from build123d import *

# Parameters (mm, degrees)
SKIZZE1_W                       = 60
SKIZZE1_H                       = 60
AUFSATZ_LINEAR_AUSTRAGEN1_DEPTH = 3
VERRUNDUNG1_R                   = 3
SKIZZE2_R                       = 1.75
SKIZZE2_R_2                     = 3.25
SKIZZE2_R_3                     = 15
SCHNITT_LINEAR_AUSTRAGEN1_DEPTH = 12


with BuildPart() as part:
    # Skizze1 → Aufsatz-Linear austragen1 (new body)
    with BuildSketch(Plane.XY):
        Rectangle(SKIZZE1_W, SKIZZE1_H)
    extrude(amount=AUFSATZ_LINEAR_AUSTRAGEN1_DEPTH)

    # Verrundung1
    verrundung1_edges = [part.edges().sort_by_distance(p)[0] for p in [
        (-30, 30, 1.5),
        (30, 30, 1.5),
        (30, -30, 1.5),
        (-30, -30, 1.5),
    ]]
    fillet(verrundung1_edges, radius=VERRUNDUNG1_R)

    # Skizze2 → Schnitt-Linear austragen1 (cut)
    with BuildSketch(Plane.XY.offset(3)):
        with Locations((-7, -24)):
            Circle(SKIZZE2_R)
        with Locations((-7, 7)):
            Circle(SKIZZE2_R)
        with Locations((24, 7)):
            Circle(SKIZZE2_R)
        with Locations((24, -24)):
            Circle(SKIZZE2_R)
        with Locations((24, 20)):
            Circle(SKIZZE2_R_2)
        with Locations((-16, 20)):
            Circle(SKIZZE2_R_2)
        with Locations((8.5, -8.5)):
            Circle(SKIZZE2_R_3)
    extrude(amount=-SCHNITT_LINEAR_AUSTRAGEN1_DEPTH, mode=Mode.SUBTRACT)


solid = part.part
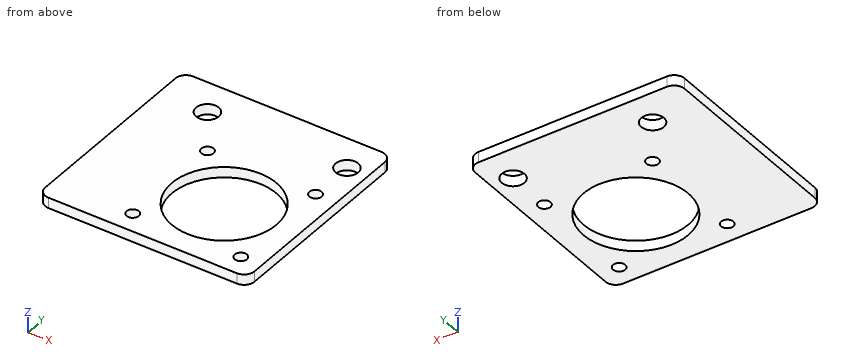
Work out the finished part from the listing and answer in its coordinate system (mm). Coordinates: 2 decimals unless noted, no trailing zeros. Write each loop counter-clockwise with the first axis right and the second up, starting at its lowest first coordinate (ties: lowest second). Pieces come first, ordered by that corner, then holes.
1. The part is cut by section D-D, the plane y = -8.5. Write down the section's boundary in (x, z), and give its area (3 significant figures).
Results list:
outline: (-30, 0) - (-6.5, 0) - (-6.5, 3) - (-30, 3) - close; (23.5, 0) - (30, 0) - (30, 3) - (23.5, 3) - close
area: 90.0 mm2
2. The part is cut by section A-A, the plane z = 2.5. Write down the section's boundary in (x, y).
Results list:
outline: (-30, -27) arc R3 ccw to (-27, -30) - (27, -30) arc R3 ccw to (30, -27) - (30, 27) arc R3 ccw to (27, 30) - (-27, 30) arc R3 ccw to (-30, 27) - close; hole circle Ø6.5 at (-16, 20); hole circle Ø3.5 at (-7, -24); hole circle Ø3.5 at (-7, 7); hole circle Ø30 at (8.5, -8.5); hole circle Ø6.5 at (24, 20); hole circle Ø3.5 at (24, -24); hole circle Ø3.5 at (24, 7)
3. The part is cut by section C-C, the plane x = 5.5. Write down the section's boundary in (y, z), and give its area (3 significant figures).
Results list:
outline: (-30, 0) - (-23.2, 0) - (-23.2, 3) - (-30, 3) - close; (6.2, 0) - (30, 0) - (30, 3) - (6.2, 3) - close
area: 91.8 mm2
4. Consider line 1 along Y through (x, z) = (24, 0.4); line 2 along Y through (x, z) = (-7, 0.6); line 3 along X through (y, z) = (21.5, 1.05). Determine where each line is inside the solid, lowest interval first.
Results list:
line 1: y = -30 to -25.75, -22.25 to 5.25, 8.75 to 16.75, 23.25 to 30
line 2: y = -30 to -25.75, -22.25 to 5.25, 8.75 to 30
line 3: x = -30 to -18.88, -13.12 to 21.12, 26.88 to 30
5. The part is cut by section B-B, the plane y = 20. Write down the section's boundary in (x, z).
Results list:
outline: (-30, 0) - (-19.25, 0) - (-19.25, 3) - (-30, 3) - close; (-12.75, 0) - (20.75, 0) - (20.75, 3) - (-12.75, 3) - close; (27.25, 0) - (30, 0) - (30, 3) - (27.25, 3) - close
